The listing builds one solid part. Answer for the finished solid, in the listing's coordinates (mm). Face numbers are marked on the shaded views. A direction names the side the tool comes from. Round coordinates to 2 decimals unless told otherwise and drop trailing zeros. Write each loop counter-clockwise with the first axis right and the second up, starting at its lowest first coordinate (ties: lowest second). Pieces come first, ordered by that corner, then holes. Notation, with made-up numbers: (3, 30.25) - (7, 30.25) arc R23 ccw to (7, 58.25) - close; hole circle Ø10 at (21, 75). An arc over 180 degrees is marked (long way). Answer as CSV lines item,"result". Start each with the question number.
Item 1: For a pull along Y with two mould halves and no side action, classify the marked faces 4, 5, 6 and 7 as pulls with the +Y half, pulls with the -Y half, needs draft (parallel to the pull), parting line crosses it, or undercut.
Item 2: Flat-ended cylindrical pins translate along their axes: pin 1 (18 mm diameter, centred on x = 6, z = -21, fed in from -Y); pin 2 (2 mm diameter, centred on x = -9, z = -23.5, fed in from +Y). Find the tip coordinate at first contact, or state that the pin passes through.
Item 3: A cutting plane is placed at C-C on x = 32. Determine the outline of the cut face in (y, z).
Item 4: A cutting plane is placed at A-A on z = -40. Determine the outline of the cut face in (x, y).
Item 5: Which of the six approach directions +Z, -Z, +X, -X, +Y, -Y give full straight-line access (tool end or side, diameter ignored) to the marked faces 1, 2 and 3?
Item 6: A cutting plane is placed at D-D on y = 20.5. Determine the outline of the cut face in (x, z), and give its area (3 significant figures).
Item 7: Straight lines are drawn through the part: line 1 along X through (y, z) = (-52, -32); line 2 along Y through (x, z) = (39, -40); line 3 along Y through (x, z) = (-43.25, -40). For each, find the intervals that lie inside material, in ascending order. Write a range as [from, to].
Item 8: A cutting plane is placed at B-B on y = -3.5. Determine the outline of the cut face in (x, z), and give its area (3 significant figures).
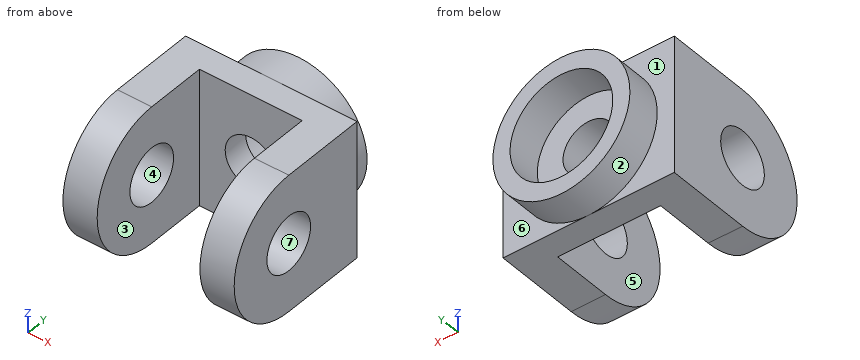
```python
from build123d import *

# Parameters (mm, degrees)
BOSS_EXTRUDE1_DEPTH = 80
BOSS_EXTRUDE2_DEPTH = 20
SKETCH3_R           = 16
CUT_EXTRUDE1_DEPTH  = 20
SKETCH4_R           = 40
SKETCH4_R_2         = 30
BOSS_EXTRUDE3_DEPTH = 20
SKETCH5_R           = 15
CUT_EXTRUDE2_DEPTH  = 131.384048104


with BuildPart() as part:
    # Sketch1 → Boss-Extrude1 (new body)
    with BuildSketch(Plane.XY):
        Polygon((30, -25), (50, -25), (50, 25), (-50, 25), (-50, -25), (-30, -25), (-30, 10), (30, 10), align=None)
    extrude(amount=-BOSS_EXTRUDE1_DEPTH)

    # Sketch2 → Boss-Extrude2 (add)
    with BuildSketch(Plane(origin=(50, 0, 0), x_dir=(0, 0, -1), z_dir=(1, 0, 0))):
        with BuildLine():
            Line((0, -25), (80, -25))
            ThreePointArc((80, -25), (40, -65), (0, -25))
        make_face()
    boss_extrude2 = extrude(amount=-BOSS_EXTRUDE2_DEPTH)

    # Sketch3 → Cut-Extrude1 (cut)
    with BuildSketch(Plane(origin=(50, 0, 0), x_dir=(0, 0, -1), z_dir=(1, 0, 0))):
        with Locations((40, -25)):
            Circle(SKETCH3_R)
    cut_extrude1 = extrude(amount=-CUT_EXTRUDE1_DEPTH, mode=Mode.SUBTRACT)

    # Mirror1: Boss-Extrude2, Cut-Extrude1 across plane
    add(boss_extrude2.mirror(Plane(origin=(0, 0, 0), x_dir=(0, 0, 1), z_dir=(1, 0, 0))))
    add(cut_extrude1.mirror(Plane(origin=(0, 0, 0), x_dir=(0, 0, 1), z_dir=(1, 0, 0))), mode=Mode.SUBTRACT)

    # Sketch4 → Boss-Extrude3 (add)
    with BuildSketch(Plane(origin=(0, 25, 0), x_dir=(1, 0, 0), z_dir=(0, 1, 0))):
        with Locations(Location((0, 40, 0), (0, 0, 270))):
            Circle(SKETCH4_R)
        with Locations(Location((0, 40, 0), (0, 0, 270))):
            Circle(SKETCH4_R_2, mode=Mode.SUBTRACT)
    extrude(amount=BOSS_EXTRUDE3_DEPTH)

    # Sketch5 → Cut-Extrude2 (cut, through all)
    with BuildSketch(Plane(origin=(0, 25, 0), x_dir=(1, 0, 0), z_dir=(0, 1, 0))):
        with Locations(Location((0, 40, 0), (0, 0, 270))):
            Circle(SKETCH5_R)
    extrude(amount=-CUT_EXTRUDE2_DEPTH, mode=Mode.SUBTRACT)


solid = part.part
```
Geometry says:
1,face 4,"undercut"
1,face 5,"needs draft"
1,face 6,"pulls with the +Y half"
1,face 7,"undercut"
2,pin 1,"stops at y = 10"
2,pin 2,"stops at y = 25"
3,outline,"(-25, -80) - (25, -80) - (25, -64) - (45, -64) - (45, -16) - (25, -16) - (25, 0) - (-25, 0) arc R40 ccw to start; hole circle Ø32 at (-25, -40)"
4,outline,"(-50, -65) - (-30, -65) - (-30, -41) - (-50, -41) - close; (-50, -9) - (-30, -9) - (-30, 10) - (-15, 10) - (-15, 25) - (-30, 25) - (-30, 45) - (-40, 45) - (-40, 25) - (-50, 25) - close; (15, 10) - (30, 10) - (30, -9) - (50, -9) - (50, 25) - (40, 25) - (40, 45) - (30, 45) - (30, 25) - (15, 25) - close; (30, -65) - (50, -65) - (50, -41) - (30, -41) - close"
5,face 1,"-X, +Y"
5,face 2,"+Y"
5,face 3,"+Z, -Z, -Y"
6,outline,"(-50, -80) - (50, -80) - (50, 0) - (-50, 0) - close; hole circle Ø30 at (0, -40)"
6,area,"7,290 mm^2"
7,line 1,"x = [-50, -30], [30, 50]"
7,line 2,"y = [-65, -41], [-9, 45]"
7,line 3,"y = [-65, -41], [-9, 25]"
8,outline,"(-50, -80) - (-30, -80) - (-30, 0) - (-50, 0) - close; (30, -80) - (50, -80) - (50, 0) - (30, 0) - close"
8,area,"3,200 mm^2"
